from build123d import *

# Parameters (mm, degrees)
SKETCH_1_W          = 58
SKETCH_1_H          = 40
EXTRUDE_1_DEPTH     = 17
SKETCH_2_R          = 1.5
CUT_EXTRUDE_1_DEPTH = 5
SKETCH_3_W          = 43
SKETCH_3_H          = 34
CUT_EXTRUDE_2_DEPTH = 0.5
SKETCH_4_R          = 3.5
SKETCH_4_R_2        = 1
EXTRUDE_2_DEPTH     = 1


with BuildPart() as part:
    # 草图1 → 凸台-拉伸1 (new body)
    with BuildSketch(Plane.XY):
        Rectangle(SKETCH_1_W, SKETCH_1_H)
    extrude(amount=EXTRUDE_1_DEPTH)

    # 草图2 → 切除-拉伸1 (cut)
    with BuildSketch(Plane.XY.offset(17)):
        with Locations((-24, -15)):
            Circle(SKETCH_2_R)
        with Locations((24, -15)):
            Circle(SKETCH_2_R)
        with Locations((-14.2, 15)):
            Circle(SKETCH_2_R)
        with Locations((14.2, 15)):
            Circle(SKETCH_2_R)
    extrude(amount=-CUT_EXTRUDE_1_DEPTH, mode=Mode.SUBTRACT)

    # 草图3 → 切除-拉伸2 (cut)
    with BuildSketch(Plane(origin=(0, 0, 0), x_dir=(-1, 0, 0), z_dir=(0, 0, -1))):
        with Locations((-4.5, 0)):
            Rectangle(SKETCH_3_W, SKETCH_3_H)
    extrude(amount=-CUT_EXTRUDE_2_DEPTH, mode=Mode.SUBTRACT)

    # 草图4 → 凸台-拉伸2 (add)
    with BuildSketch(Plane.XY.offset(17)):
        with Locations((0, 10)):
            Circle(SKETCH_4_R)
        with Locations((0, 10)):
            Circle(SKETCH_4_R_2, mode=Mode.SUBTRACT)
    extrude(amount=EXTRUDE_2_DEPTH)


solid = part.part
Model file for the job. Use its own axes, mm. A direction names the side the tool comes from. Give positions to 0.01 mm unless a question says otherwise; leave off trailing zeros. Order: outer loops, then holes, each group sorted by start corner. A loop starts at its lowest first (then second) coordinate and runs counter-clockwise, first axis right, second up. Notation, with made-up numbers: M 9.25,-5 L 42.25,-5 A33 cw 42.25,28 Z; hole C 30.25,-37.75 d4. An arc over 180 degrees is marked long. Put each result on its own line as item: value. Start each with the question number.
(1) Drill centre lines: L1, parallel to Y at x = -14.2, z = 14.7; L2, parallel to Y at x = -24, z = 15.55; L3, parallel to Z at x = -10, y = 8. Where is each one in solid material? Low to high. Write a range as [from, to].
(2) Band-saw the part on B-B on x = 0. Give the cut face in (y, z), then the cut area to 3 significant figures.
(3) Band-saw the part on A-A on y = 15. Give the cut face in (x, z), then the cut area to 4 significant figures.
(4) Band-saw the part on D-D on y = 4.5. Give the cut face in (x, z).
(5) Band-saw the part on C-C on x = 20. Give the cut face in (y, z), then the cut area to 3 significant figures.
(6) Tool access for faces 1 (the face through (5, 0, 0.5)), 2 (the face through (0, -20, 8)), 3 (the face through (0, 10, 17)): list every direction of +Z, -Z, +X, -X, +Y, -Y with a clear straight run to the whole face (end or side of a thin tool).
(7) Pin check, flat tips, straight feed: pin 1 Ø2 at (x, y) = (-21, -3.5) entering from +Z; pin 2 Ø1.8 at (x, y) = (-14.2, 15) entering from +Z; pin 3 Ø10 at (x, y) = (4, -0.5) entering from -Z. Stop position of each tip, or through.
(8) Pull direction X, two halves, no side cores. Call faces 4 (the face through (-0.759, 6.583, 17.493)), 5 (the face through (-12.814, 14.425, 14.535)), 6 (the face through (-20, 0, 0)), 7 (the face through (-29, 0, 8)): released by +X, released by -X, zero draft, split by the parting line, or undercut.
Results below:
1. L1: y = [-20, 13.5], [16.5, 20]
1. L2: y = [-20, -16.5], [-13.5, 20]
1. L3: z = [0.5, 17]
2. outline: M -20,0 L -17,0 L -17,0.5 L 17,0.5 L 17,0 L 20,0 L 20,17 L 13.5,17 L 13.5,18 L 11,18 L 11,17 L 9,17 L 9,18 L 6.5,18 L 6.5,17 L -20,17 Z
2. area: 668 mm2
3. outline: M -29,0 L -17,0 L -17,0.5 L 26,0.5 L 26,0 L 29,0 L 29,17 L 15.7,17 L 15.7,12 L 12.7,12 L 12.7,17 L -12.7,17 L -12.7,12 L -15.7,12 L -15.7,17 L -29,17 Z
3. area: 934.5 mm2
4. outline: M -29,0 L -17,0 L -17,0.5 L 26,0.5 L 26,0 L 29,0 L 29,17 L -29,17 Z
5. outline: M -20,0 L -17,0 L -17,0.5 L 17,0.5 L 17,0 L 20,0 L 20,17 L -20,17 Z
5. area: 663 mm2
6. face 1: -Z
6. face 2: +Z, -Z, +X, -X, -Y
6. face 3: +Z
7. pin 1: stops at z = 17
7. pin 2: stops at z = 12
7. pin 3: stops at z = 0.5
8. face 4: split by the parting line
8. face 5: undercut
8. face 6: zero draft
8. face 7: released by -X
